Read the model definition and answer for the solid it produces. Units are mm, in the model's axes. Coordinates: 2 decimals unless noted, no trailing zeros. Loops run counter-clockwise (first coordinate to the right, second up) from the corner with the lowest first, then second, coordinate; pieces in that order, holes last. Notation, with made-up numbers: (1, 11.25) - (17, 11.25) arc R20 ccw to (17, 26.25) - close; hole circle Ø7 at (63.5, 81.5). An arc over 180 degrees is marked (long way). Use one line per item in the form item = value.
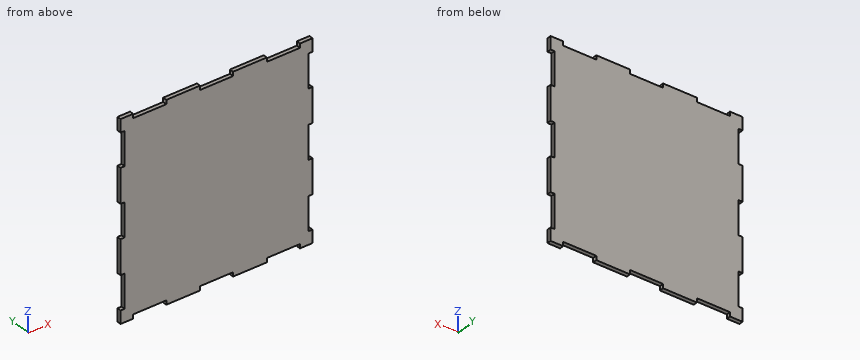
from build123d import *

# Parameters (mm, degrees)
SKETCH1_W                 = 150
SKETCH1_H                 = 150
BOSS_EXTRUDE1_DEPTH       = 3.18
SKETCH6_W                 = 12.9
SKETCH6_H                 = 3.18
SKETCH6_W_2               = 25.8
CUT_EXTRUDE1_DEPTH        = 10
MIRROR2_COPY_1_SKETCH_W   = 12.9
MIRROR2_COPY_1_SKETCH_H   = 3.18
MIRROR2_COPY_1_SKETCH_W_2 = 25.8
MIRROR2_COPY_1_DEPTH      = 10
MIRROR3_COPY_1_SKETCH_W   = 12.9
MIRROR3_COPY_1_SKETCH_H   = 3.18
MIRROR3_COPY_1_SKETCH_W_2 = 25.8
MIRROR3_COPY_1_DEPTH      = 10
MIRROR4_COPY_1_SKETCH_W   = 12.9
MIRROR4_COPY_1_SKETCH_H   = 3.18
MIRROR4_COPY_1_SKETCH_W_2 = 25.8
MIRROR4_COPY_1_DEPTH      = 10
MIRROR4_COPY_2_SKETCH_W   = 12.9
MIRROR4_COPY_2_SKETCH_H   = 3.18
MIRROR4_COPY_2_SKETCH_W_2 = 25.8
MIRROR4_COPY_2_DEPTH      = 10
MIRROR4_COPY_3_SKETCH_W   = 12.9
MIRROR4_COPY_3_SKETCH_H   = 3.18
MIRROR4_COPY_3_SKETCH_W_2 = 25.8
MIRROR4_COPY_3_DEPTH      = 10


with BuildPart() as part:
    # Sketch1 → Boss-Extrude1 (new body)
    with BuildSketch(Plane(origin=(0, 0, 0), x_dir=(1, 0, 0), z_dir=(0, 1, 0))):
        Rectangle(SKETCH1_W, SKETCH1_H)
    extrude(amount=BOSS_EXTRUDE1_DEPTH)

    # Sketch6 → Cut-Extrude1 (cut)
    with BuildSketch(Plane.XZ):
        with Locations((-6.45, 73.41)):
            Rectangle(SKETCH6_W, SKETCH6_H)
        with Locations((-52.2, 73.41)):
            Rectangle(SKETCH6_W_2, SKETCH6_H)
    cut_extrude1 = extrude(amount=-CUT_EXTRUDE1_DEPTH, mode=Mode.SUBTRACT)

    # Mirror1: Cut-Extrude1 across plane
    add(cut_extrude1.mirror(Plane(origin=(0, 0, 0), x_dir=(0, 0, 1), z_dir=(1, 0, 0))), mode=Mode.SUBTRACT)

    # Mirror2: Cut-Extrude1 across plane
    add(cut_extrude1.mirror(Plane.XY), mode=Mode.SUBTRACT)

    # Mirror2 copy 1 sketch → Mirror2 copy 1 (cut)
    with BuildSketch(Plane(origin=(0, 0, 0), x_dir=(-1, 0, 0), z_dir=(0, -1, 0))):
        with Locations((-6.45, 73.41)):
            Rectangle(MIRROR2_COPY_1_SKETCH_W, MIRROR2_COPY_1_SKETCH_H)
        with Locations((-52.2, 73.41)):
            Rectangle(MIRROR2_COPY_1_SKETCH_W_2, MIRROR2_COPY_1_SKETCH_H)
    extrude(amount=-MIRROR2_COPY_1_DEPTH, mode=Mode.SUBTRACT)

    # Mirror3: Cut-Extrude1 across plane
    add(cut_extrude1.mirror(Plane(origin=(0, 0, 0), x_dir=(-0.707106781, 0, 0.707106781), z_dir=(0.707106781, 0, 0.707106781))), mode=Mode.SUBTRACT)

    # Mirror3 copy 1 sketch → Mirror3 copy 1 (cut)
    with BuildSketch(Plane(origin=(0, 0, 0), x_dir=(0, 0, 1), z_dir=(0, -1, 0))):
        with Locations((-6.45, 73.41)):
            Rectangle(MIRROR3_COPY_1_SKETCH_W, MIRROR3_COPY_1_SKETCH_H)
        with Locations((-52.2, 73.41)):
            Rectangle(MIRROR3_COPY_1_SKETCH_W_2, MIRROR3_COPY_1_SKETCH_H)
    extrude(amount=-MIRROR3_COPY_1_DEPTH, mode=Mode.SUBTRACT)

    # Mirror4 copy 1 sketch → Mirror4 copy 1 (cut)
    with BuildSketch(Plane(origin=(0, 0, 0), x_dir=(0, 0, -1), z_dir=(0, -1, 0))):
        with Locations((-6.45, 73.41)):
            Rectangle(MIRROR4_COPY_1_SKETCH_W, MIRROR4_COPY_1_SKETCH_H)
        with Locations((-52.2, 73.41)):
            Rectangle(MIRROR4_COPY_1_SKETCH_W_2, MIRROR4_COPY_1_SKETCH_H)
    extrude(amount=-MIRROR4_COPY_1_DEPTH, mode=Mode.SUBTRACT)

    # Mirror4 copy 2 sketch → Mirror4 copy 2 (cut)
    with BuildSketch(Plane(origin=(0, 0, 0), x_dir=(0, 0, 1), z_dir=(0, -1, 0))):
        with Locations((-6.45, -73.41)):
            Rectangle(MIRROR4_COPY_2_SKETCH_W, MIRROR4_COPY_2_SKETCH_H)
        with Locations((-52.2, -73.41)):
            Rectangle(MIRROR4_COPY_2_SKETCH_W_2, MIRROR4_COPY_2_SKETCH_H)
    extrude(amount=-MIRROR4_COPY_2_DEPTH, mode=Mode.SUBTRACT)

    # Mirror4 copy 3 sketch → Mirror4 copy 3 (cut)
    with BuildSketch(Plane(origin=(0, 0, 0), x_dir=(-1, 0, 0), z_dir=(0, -1, 0))):
        with Locations((-6.45, -73.41)):
            Rectangle(MIRROR4_COPY_3_SKETCH_W, MIRROR4_COPY_3_SKETCH_H)
        with Locations((-52.2, -73.41)):
            Rectangle(MIRROR4_COPY_3_SKETCH_W_2, MIRROR4_COPY_3_SKETCH_H)
    extrude(amount=-MIRROR4_COPY_3_DEPTH, mode=Mode.SUBTRACT)


solid = part.part
Item 1: The part is cut by section A-A on z = 3.5. Give the vertices of the cut face in (x, y), plus the area to 3 significant figures.
Results below:
outline = (-71.82, 0) - (71.82, 0) - (71.82, 3.18) - (-71.82, 3.18) - close
area = 457 mm²
Item 2: Find the intervals of material crossed by L1, parallel to Z at x = 58.5, y = 0.3, in increasing order.
Results below:
L1 = -71.82 to 71.82
Item 3: Each of these flat-tipped pins is pushed along its axis until it touches: P1, Ø1.6, axis at x = -0.5, y = 1.5, coming from the +Z side; P2, Ø1, axis at y = 1.5, z = 47, coming from the -X side. Where does it stop, or does it pass through?
Results below:
P1 = 71.82
P2 = -71.82
Item 4: The part is cut by section B-B on x = -52. Give the vertices of the cut face in (y, z).
Results below:
outline = (0, -71.82) - (3.18, -71.82) - (3.18, 71.82) - (0, 71.82) - close
